Input: dimensioned drawing with shaded views. Units: mm. Origin: part minimum x, y, z. A direction names the side the tool comes from. Round coordinates to 2 decimals unless told otherwise and drop trailing zeros. Loops run counter-clockwise (first coordinate to the right, second up) from the corner with the lowest first, then second, coordinate; pieces in that order, holes last. Notation, with made-up numbers: (87, -21) - (107, -21) arc R11 ccw to (107, -4) - close; hole circle Ø8 at (-37.75, -19). An arc over 180 degrees is marked (long way). One line per question, with ' | ' between items. Start each with the question number.
Item 1: Section B-B, the plane x = 5.25. Return loops of the section in (y, z).
Item 2: Section C-C, the plane z = 5.5. Return loops of the section in (x, y) (3 decimals), plus the area to 3 significant figures.
Item 3: Draft query along Z for the marked faces 6, 7, 8 and 9. Return one class per face: pulls with the +Z half, pulls with the -Z half, needs draft (parallel to the pull), parting line crosses it, or undercut.
Item 4: Set-up query: the marked faces 1, 2, 3, 4 and 5. Return all of +Z, -Z, +X, -X, +Y, -Y with unobstructed straight access to the full face (end or side cutting, diameter ignored); none if empty.
Item 5: Section D-D, the plane y = 15.5. Return loops of the section in (x, z), plus the area to 3 significant figures.
Item 6: Section A-A, the plane y = 9.5. Return loops of the section in (x, z) (3 decimals), plus the area to 3 significant figures.
Item 7: Material intervals for line 1 along X through (y, z) = (13.5, 8.5); line 2 along Y through (x, z) = (4.75, 1.75); line 3 along Y through (x, z) = (9.5, 3), sorted ascending.
Item 8: First-contact query: pin 1 (1.5 mm diameter, centred on x = 3.5, y = 14.5, fed in from +Z); pin 2 (4.5 mm diameter, centred on y = 15, z = 4, fed in from -X); pin 3 (3.5 mm diameter, centred on x = 3, z = 5.5, fed in from +Y); pin 4 (6.5 mm diameter, centred on x = 3, z = 6.5, fed in from +Y). Flat tips, straight axial feed; report the tip coordinate or a pass-through.
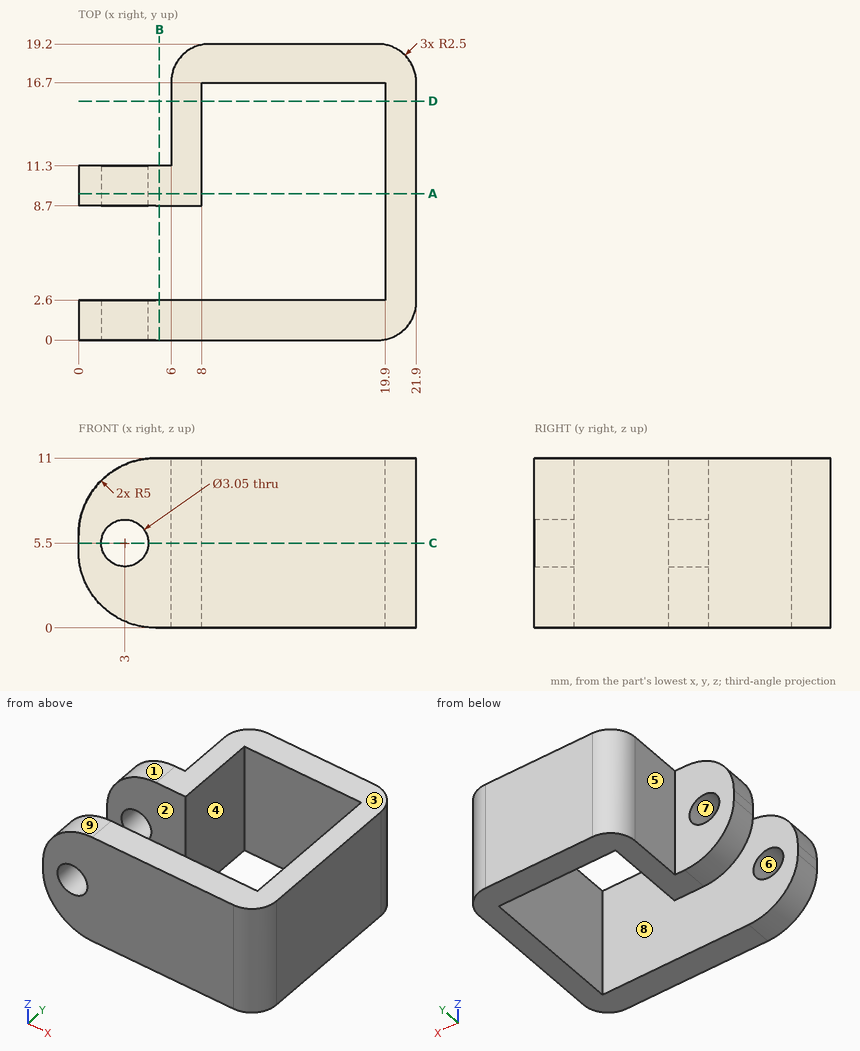
Return value:
1) outline: (0, 0) - (2.6, 0) - (2.6, 11) - (0, 11) - close; (8.7, 0) - (11.3, 0) - (11.3, 11) - (8.7, 11) - close
2) outline: (0, 0) - (1.475, 0) - (1.475, 2.6) - (0, 2.6) - close; (0, 8.7) - (1.475, 8.7) - (1.475, 11.3) - (0, 11.3) - close; (4.525, 0) - (19.4, 0) arc R2.5 ccw to (21.9, 2.5) - (21.9, 16.7) arc R2.5 ccw to (19.4, 19.2) - (8.5, 19.2) arc R2.5 ccw to (6, 16.7) - (6, 11.3) - (4.525, 11.3) - (4.525, 8.7) - (8, 8.7) - (8, 16.7) - (19.9, 16.7) - (19.9, 2.6) - (4.525, 2.6) - close | area: 137 mm2
3) face 6: undercut | face 7: undercut | face 8: needs draft | face 9: pulls with the +Z half
4) face 1: +Z, -X, +Y, -Y | face 2: +Z, -Z, -X | face 3: +Z, +X, -X, +Y, -Y | face 4: +Z, -Z | face 5: +Z, -Z, -X, +Y
5) outline: (6, 0) - (8, 0) - (8, 11) - (6, 11) - close; (19.9, 0) - (21.9, 0) - (21.9, 11) - (19.9, 11) - close | area: 44.0 mm2
6) outline: (0, 5) arc R5 ccw to (5, 0) - (8, 0) - (8, 11) - (5, 11) arc R5 ccw to (0, 6) - close; (19.9, 0) - (21.9, 0) - (21.9, 11) - (19.9, 11) - close; hole circle Ø3.05 at (3, 5.5) | area: 92.0 mm2
7) line 1: 6 to 8, 19.9 to 21.9 | line 2: 0 to 2.6, 8.7 to 11.3 | line 3: 0 to 2.6, 16.7 to 19.2
8) pin 1: through | pin 2: x = 6 | pin 3: y = 11.3 | pin 4: y = 17.79
